Solid Edge part; units mm, degrees
sketch "Sketch1" plane through (0, 0, 0) normal (0, 0, 1) x (1, 0, 0)
  line L0 (0, 0) -> (100, 0)
  line L1 (100, 0) -> (100, 50)
  circle A0 centre (101, 25) radius 14.3
  line L2 (100, 50) -> (0, 50)
  line L3 (0, 50) -> (0, 0)
extrude "Protrusion1" add sketch "Sketch1" along normal blind 15
hole "Bohrung_1" at (100, 5.3675, 7.5) direction (-1, 0, 0) diameter 3.242 depth 15 thread major 4 thread length 10
hole "Hole1" at (100, 44.6325, 7.5) direction (-1, 0, 0) diameter 3.242 depth 15 thread major 4 thread length 10
hole "Bohrung_3" at (10, 25, 15) direction (0, 0, -1) diameter 6.5 end through all
hole "Hole2" at (45, 25, 15) direction (0, 0, -1) diameter 6.5 end through all
fillet "Verrundung_2" radius 0.5 6 edges at (0, 50, 7.5) (0, 0, 7.5) (100, 0, 7.5) (100, 10.735, 7.5) (100, 39.265, 7.5) (100, 50, 7.5)
Design review of the part built by this model. Coordinates are the model's own, in mm. A direction names the side the tool comes from. Give positions to 0.01 mm unless a question says otherwise; leave off trailing zeros. Loops run counter-clockwise (first coordinate to the right, second up) from the corner with the lowest first, then second, coordinate; pieces in that order, holes last. Notation, with made-up numbers: (78.5, 65) - (136.5, 65) arc R27 cw to (136.5, 82) - close; hole circle Ø6 at (55.5, 46.25). An arc over 180 degrees is marked (long way). Use CSV: the item, a comma, the result in double quotes. Start each with the question number.
1. Wall thickness on L1, parallel to Y at x = 10, z = 11.5; L2, parallel to Y at x = 95.25, z = 7.5; L3, parallel to Y at x = 93.5, z = 7.5: over which ranges is each line inside the solid? List them lowest first.
2. Add section D-D (y = 35). State the section outline as (x, z) points.
3. Add section A-A (z = 7.5). State the section outline as (x, y) points.
4. Draft analysis for pull direction Z (two halves, no side actions). For faces 3 (the cylindrical face through (41.827, 25.705, 7.605)), 4 (the flat face through (85, 45, 8)), 5 (the cylindrical face through (92.4, 6.35, 8.79)), 6 (the flat face through (49, 25, 15)), state which applies: released by +Z, released by -Z, zero draft, split by the parting line, or undercut.
5. Add section C-C (y = 25). State the section outline as (x, z) points, plus the area to 3 significant figures.
6. Insertion check: P1, Ø5, axis at y = 20.5, z = 11, coming from the +X side; P2, Ø4, axis at x = 45, y = 25, coming from the -Z side. Each pin has a flat end and moves straight along its axis. Give the tip position at first contact, or say it passes through.
7. Machinability: for faces 1 (the flat face through (49, 0, 7)), 2 (the cylindrical face through (92.395, 43.025, 7.711)), which of the approach directions +Z, -Z, +X, -X, +Y, -Y give a long, thin tool a straight path to every point of the face, cutting with its end or side? Answer none if there is none.
8. Add section B-B (x = 10). State the section outline as (y, z) points, plus the area to 4 significant figures.
Results found:
1,L1,"y = 0 to 21.75, 28.25 to 50"
1,L2,"y = 0 to 3.75, 6.99 to 11.91, 38.09 to 43.01, 46.25 to 50"
1,L3,"y = 0 to 3.75, 6.99 to 12.82, 37.18 to 43.01, 46.25 to 50"
2,outline,"(0, 0) - (90.78, 0) - (90.78, 15) - (0, 15) - close"
3,outline,"(0, 0.5) arc R0.5 ccw to (0.5, 0) - (99.5, 0) arc R0.5 ccw to (100, 0.5) - (100, 3.75) - (85, 3.75) - (85, 6.99) - (100, 6.99) - (100, 10.28) arc R0.5 ccw to (99.55, 10.77) arc R14.3 cw to (99.55, 39.23) arc R0.5 ccw to (100, 39.72) - (100, 43.01) - (85, 43.01) - (85, 46.25) - (100, 46.25) - (100, 49.5) arc R0.5 ccw to (99.5, 50) - (0.5, 50) arc R0.5 ccw to (0, 49.5) - close; hole circle Ø6.5 at (10, 25); hole circle Ø6.5 at (45, 25)"
4,face 3,"zero draft"
4,face 4,"undercut"
4,face 5,"undercut"
4,face 6,"released by +Z"
5,outline,"(0, 0) - (6.75, 0) - (6.75, 15) - (0, 15) - close; (13.25, 0) - (41.75, 0) - (41.75, 15) - (13.25, 15) - close; (48.25, 0) - (86.7, 0) - (86.7, 15) - (48.25, 15) - close"
5,area,"1,110 mm²"
6,P1,"stops at x = 88.53"
6,P2,"passes through"
7,face 1,"+Z, -Z, +X, -X, -Y"
7,face 2,"+X"
8,outline,"(0, 0) - (21.75, 0) - (21.75, 15) - (0, 15) - close; (28.25, 0) - (50, 0) - (50, 15) - (28.25, 15) - close"
8,area,"652.5 mm²"
